Could you check a few things on this drawing? It's one solid part, dimensions in mm from its lowest x, y, z. Coordinates: 2 decimals unless noted, no trailing zeros. Write each loop counter-clockwise with the first axis right and the second up, starting at its lowest first coordinate (ties: lowest second). Pieces come first, ordered by that corner, then holes. Notation, with made-up numbers: (50.25, -24.5) - (98.25, -24.5) arc R15 ccw to (98.25, -13.5) - close; hole circle Ø2 at (-18, 25). An arc over 180 degrees is marked (long way). Answer as a JSON object with one key per item and string values. Group by question number.
1) Will these pins go through, and if not, where does the flat tip stop? pin 1 Ø5.5 at (x, y) = (261.74, 211.39) entering from +Z; pin 2 Ø2 at (y, z) = (70.5, 3.5) entering from -X.
2) Please list where these lines run through material, in increasing order: line 1 along Y through (x, z) = (144, 4.75) (1 decimal); line 2 along X through (y, z) = (197.5, 4.5) (1 decimal); line 3 along Y through (x, z) = (130, 3.25).
3) If we section it at B-B (x = 232): Write out the boundary of the cut face in (y, z) (1 decimal).
4) If we section it at A-A (y = 105): Write out the boundary of the cut face in (x, z) (1 decimal), plus the area to 3 significant figures.
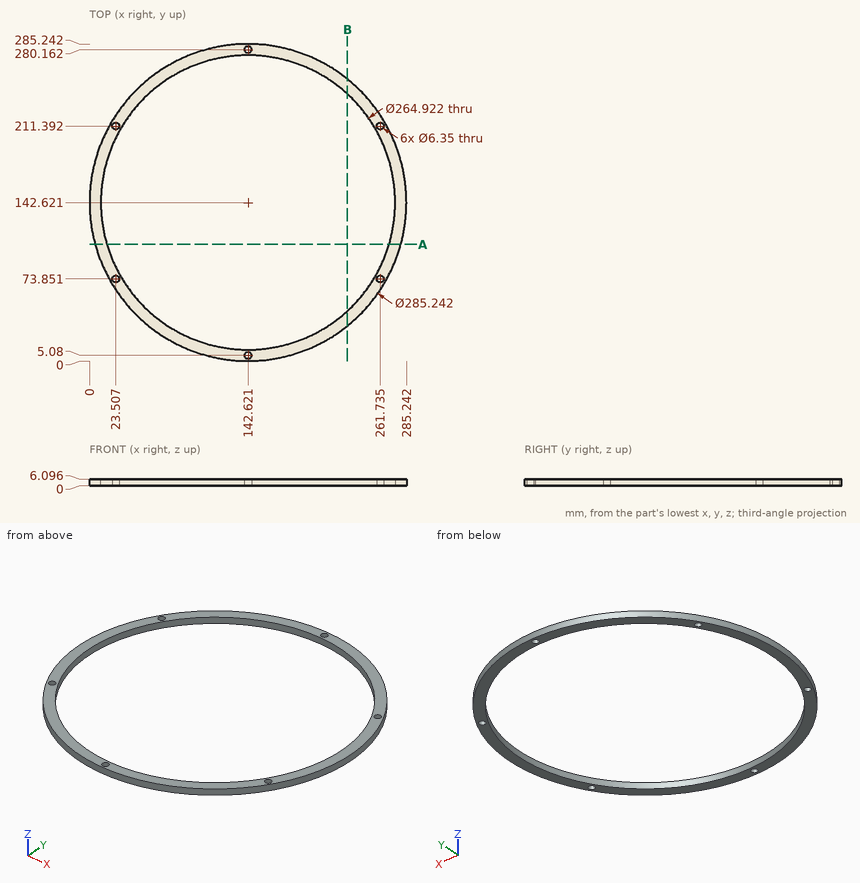
Here are the results:
{
 "1": {"pin 1": "passes through", "pin 2": "stops at x = 19"},
 "2": {"line 1": "y = 0 to 2.2, 7.9 to 10.2, 275.1 to 277.3, 283 to 285.2", "line 2": "x = 11 to 22.1, 263.2 to 274.3", "line 3": "y = 0.56 to 10.76, 274.48 to 284.68"},
 "3": {"outline": "(31.5, 0) - (44.9, 0) - (44.9, 6.1) - (31.5, 6.1) - close; (240.4, 0) - (253.8, 0) - (253.8, 6.1) - (240.4, 6.1) - close"},
 "4": {"outline": "(5.1, 0) - (15.6, 0) - (15.6, 6.1) - (5.1, 6.1) - close; (269.6, 0) - (280.2, 0) - (280.2, 6.1) - (269.6, 6.1) - close", "area": "129 mm²"}
}
